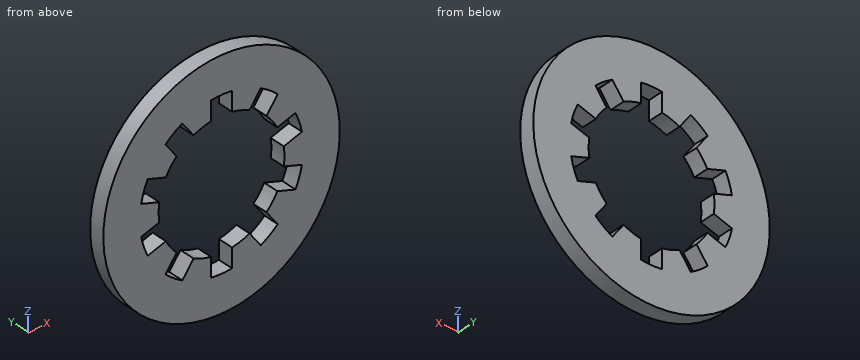
```python
from build123d import *

# Parameters (mm, degrees)
SKETCH1_R          = 9.4996
SKETCH1_R_2        = 5.0546
EXTRUDE1_DEPTH     = 1.27
CUT_EXTRUDE1_DEPTH = 14.494358092
CIRPATTERN1_COUNT  = 10


with BuildPart() as part:
    # Sketch1 → Extrude1 (new body)
    with BuildSketch(Plane(origin=(0, 0, 0), x_dir=(1, 0, 0), z_dir=(0, 1, 0))):
        with Locations(Location((0, 0, 0), (0, 0, 270))):
            Circle(SKETCH1_R)
        with Locations(Location((0, 0, 0), (0, 0, 270))):
            Circle(SKETCH1_R_2, mode=Mode.SUBTRACT)
    extrude(amount=EXTRUDE1_DEPTH)

    # Sketch2 → Cut-Extrude1 (cut, through all)
    with BuildSketch(Plane(origin=(0, 1.27, 0), x_dir=(-1, 0, 0), z_dir=(0, 1, 0))):
        with BuildLine():
            Line((-0.842433333, 6.516754118), (-0.842433333, 4.983902812))
            ThreePointArc((-0.842433333, 4.983902812), (0, 5.0546), (0.842433333, 4.983902812))
            Line((0.842433333, 4.983902812), (0.842433333, 6.516754118))
            ThreePointArc((0.842433333, 6.516754118), (0, 6.57098), (-0.842433333, 6.516754118))
        make_face()
    cut_extrude1 = extrude(amount=-CUT_EXTRUDE1_DEPTH, mode=Mode.SUBTRACT)

    # CirPattern1: Cut-Extrude1 ×10 about axis
    cirpattern1_axis = Axis((0, 0, 0), (0, 1, 0))
    for i in range(1, CIRPATTERN1_COUNT):
        add(cut_extrude1.rotate(cirpattern1_axis, i * 360 / CIRPATTERN1_COUNT), mode=Mode.SUBTRACT)


solid = part.part
```
Source: CAD feature listing. Evaluate the final solid. Frame: model axes, mm. Round coordinates to 2 decimals unless told otherwise and drop trailing zeros. Write each loop counter-clockwise with the first axis right and the second up, starting at its lowest first coordinate (ties: lowest second). Pieces come first, ordered by that corner, then holes. Notation, with made-up numbers: M 2,-14.5 L 19,-14.5 A3 cw 19,-10.5 Z; hole C 74,37.25 d2. An arc over 180 degrees is marked long. Use CSV: the item, a comma, the result in double quotes. Start each with the question number.
Q1. Cut plane D-D on z = 7.5. Output: boundary loops of the cut face in (x, y).
Q2. Cut plane A-A on z = 0. Output: boundary loops of the cut face in (x, y).
Q3. Line query: line 1 (Z direction, x = 5.25, y = 0.3); line 2 (Z direction, x = 0.5, y = 1.1); line 3 (Z direction, x = -2, y = 0.45). Output: solid intervals per line, ascending. Write a range as from..to.
Q4. Cut plane B-B on x = 0. Output: boundary loops of the cut face in (y, z).
Q5. First-contact query: P1, Ø3, axis at x = 0, z = 5, coming from the +Y side; P2, Ø0.6, axis at y = 0.5, z = -6, coming from the -X side. Flat tips, straight axial feed; report the tip coordinate or a pass-through.
Q6. Cut plane C-C on x = 4. Output: boundary loops of the cut face in (y, z), plus the area to 3 significant figures.
Results found:
1,outline,"M -5.83,0 L 5.83,0 L 5.83,1.27 L -5.83,1.27 Z"
2,outline,"M -9.5,0 L -5.05,0 L -5.05,1.27 L -9.5,1.27 Z; M 5.05,0 L 9.5,0 L 9.5,1.27 L 5.05,1.27 Z"
3,line 1,"-7.92..-2.59, -0.82..0.82, 2.59..7.92"
3,line 2,"-9.49..-6.55, 6.55..9.49"
3,line 3,"-9.29..-4.64, 4.64..9.29"
4,outline,"M 0,-9.5 L 1.27,-9.5 L 1.27,-6.57 L 0,-6.57 Z; M 0,6.57 L 1.27,6.57 L 1.27,9.5 L 0,9.5 Z"
5,P1,"y = 1.27"
5,P2,"x = -7.6"
6,outline,"M 0,-8.62 L 1.27,-8.62 L 1.27,-5.21 L 0,-5.21 Z; M 0,-4.07 L 1.27,-4.07 L 1.27,-3.09 L 0,-3.09 Z; M 0,3.09 L 1.27,3.09 L 1.27,4.07 L 0,4.07 Z; M 0,5.21 L 1.27,5.21 L 1.27,8.62 L 0,8.62 Z"
6,area,"11.1 mm^2"
